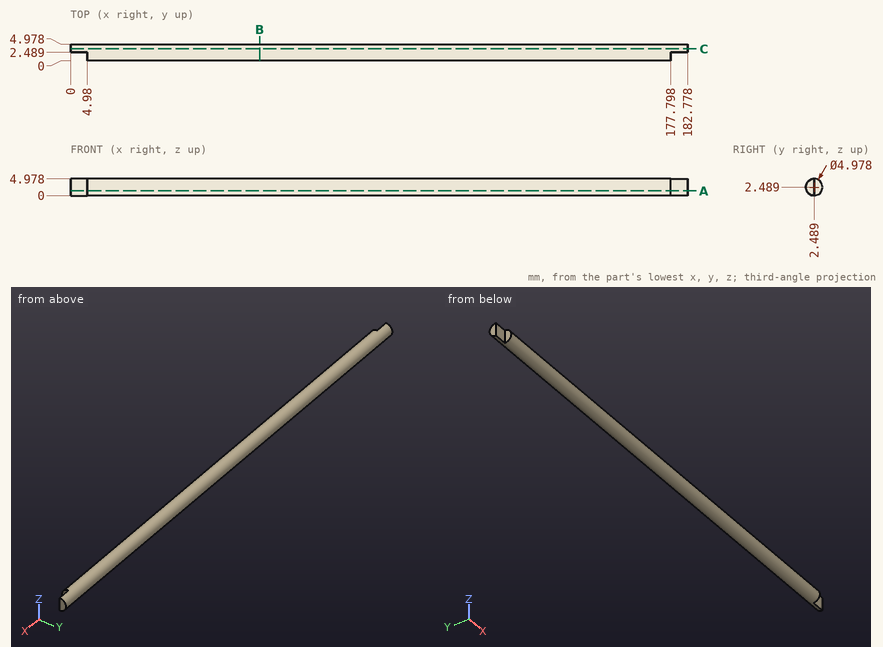
The figure shows three views and two pictorial views of one solid part (mm, origin at its lowest corner). Answer the questions. Round coordinates to 2 decimals unless told otherwise and drop trailing zeros. Write each loop counter-clockwise with the first axis right and the second up, starting at its lowest first coordinate (ties: lowest second). Pieces come first, ordered by that corner, then holes. Notation, with made-up numbers: (27, 0.5) -> (32, 0.5) arc R32 ccw to (32, 34.5) -> close; hole circle Ø8 at (-17.5, -10.5). An arc over 180 degrees is marked (long way). Write each question's results on one line, items separated by ' | '.
Q1. Straight lines are drawn through the part: line 1 along X through (y, z) = (1.9, 3.8); line 2 along Z through (x, y) = (72, 2.7); line 3 along Y through (x, z) = (133, 4.15) (1 decimal). For each, find the intervals that lie inside material, in ascending order. Write a range as [from, to].
Data:
line 1: [4.98, 177.8] | line 2: [0.01, 4.97] | line 3: [0.6, 4.3]
Q2. Flat-ended cylindrical pins translate along their axes: P1, Ø0.7, axis at y = 1, z = 2, coming from the +X side; P2, Ø1.5, axis at y = 1.5, z = 1.5, coming from the -X side; P3, Ø1.5, axis at x = 181, z = 3.5, coming from the -Y side. Find the tip coordinate at first contact, or state that the pin passes through.
Data:
P1: x = 177.8 | P2: x = 4.98 | P3: y = 2.49
Q3. Section A-A, the plane z = 1.4 is taken. Write down the section's boundary in (x, y).
Data:
outline: (0, 2.49) -> (4.98, 2.49) -> (4.98, 0.25) -> (177.8, 0.25) -> (177.8, 2.49) -> (182.78, 2.49) -> (182.78, 4.73) -> (0, 4.73) -> close
Q4. Section B-B, the plane x = 56 is taken. Write down the section's boundary in (y, z), then the cut area to 3 significant figures.
Data:
outline: circle Ø4.98 at (2.49, 2.49) | area: 19.5 mm^2
Q5. Section C-C, the plane y = 3.5 is taken. Write down the section's boundary in (x, z) (1 decimal).
Data:
outline: (0, 0.2) -> (182.8, 0.2) -> (182.8, 4.8) -> (0, 4.8) -> close
